Input: dimensioned drawing with shaded views. Units: mm. Origin: part minimum x, y, z. A direction names the side the tool comes from. Give positions to 0.01 mm unless a question says otherwise; leave off trailing zeros. Loops run counter-clockwise (first coordinate to the right, second up) from the corner with the lowest first, then second, coordinate; pieces in that order, holes last.
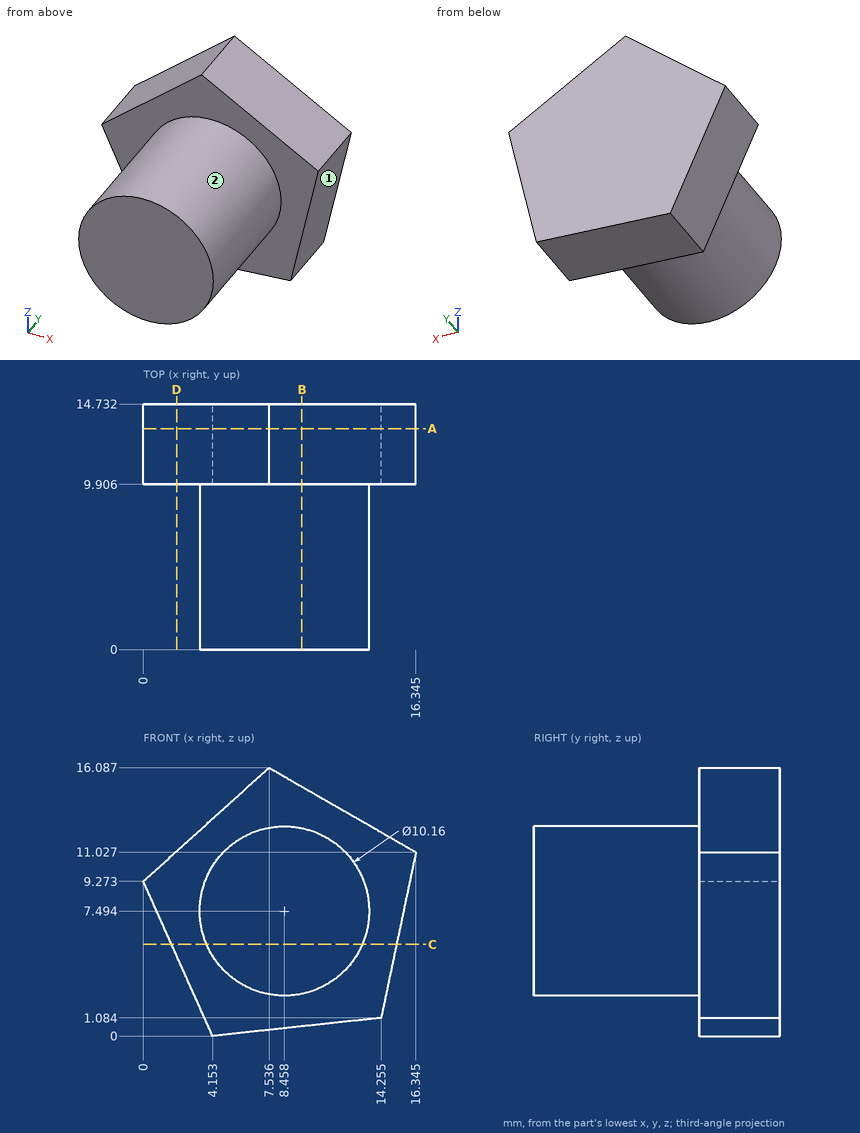
(1) Section C-C, the plane z = 5.5. Return the cut outline in (x, y) (1 decimal), then the cut area to 3 significant figures.
A:
outline: (1.7, 9.9) - (3.8, 9.9) - (3.8, 0) - (13.1, 0) - (13.1, 9.9) - (15.2, 9.9) - (15.2, 14.7) - (1.7, 14.7) - close
area: 158 mm2
(2) Section B-B, the plane x = 9.5. Return the cut outline in (y, z).
A:
outline: (0, 2.52) - (9.91, 2.52) - (9.91, 0.57) - (14.73, 0.57) - (14.73, 14.96) - (9.91, 14.96) - (9.91, 12.47) - (0, 12.47) - close
(3) First-contact query: pin 1 (8 mm diameter, centred on x = 9, y = 5.5, fed in from -Z); pin 2 (1 mm diameter, centred on y = 10.5, z = 14, fed in from +X). Flat tips, straight axial feed; report the tip coordinate or a pass-through.
A:
pin 1: stops at z = 2.41
pin 2: stops at x = 12.04
(4) Ray query, line 1 along Y through (x, z) = (15, 9.5); line 2 along Z through (x, y) = (9.25, 6.25); line 3 along X through (y, z) = (1, 10) (1 decimal). Return the intervals inside material, ascending.
A:
line 1: y = 9.91 to 14.73
line 2: z = 2.48 to 12.51
line 3: x = 4 to 12.9
(5) Section A-A, the plane y = 13.25. Return the cut outline in (x, z) (1 decimal), then the cut area to 3 significant figures.
A:
outline: (0, 9.3) - (4.2, 0) - (14.3, 1.1) - (16.3, 11) - (7.5, 16.1) - close
area: 178 mm2
(6) Reachability of the marked faces 1 and 2 from +Z, -Z, +X, -X, +Y, -Y: full face, straight path, thin tool, end or side. Return the list, or none.
A:
face 1: -Z, +X, +Y, -Y
face 2: -Y
(7) Section D-D, the plane x = 2. Return the cut outline in (y, z), then the cut area to 3 significant figures.
A:
outline: (9.91, 4.81) - (14.73, 4.81) - (14.73, 11.08) - (9.91, 11.08) - close
area: 30.3 mm2
